Work out the finished part from the listing and answer in its coordinate system (mm). A direction names the side the tool comes from. Round coordinates to 2 decimals unless told otherwise and drop trailing zeros. Loops run counter-clockwise (first coordinate to the right, second up) from the corner with the lowest first, then second, coordinate; pieces in that order, holes last. Notation, with made-up numbers: (28.5, 24) - (40.5, 24) arc R28 ccw to (40.5, 44) - close; hole circle Ø1 at (20.25, 3.5). An arc over 180 degrees is marked (long way). Answer as CSV lines item,"result". Start each with the question number.
Q1. Each of these flat-tipped pins is pushed along its axis until it touches: pin 1 Ø1.1 at (y, z) = (11, -8) entering from +X; pin 2 Ø1.2 at (x, z) = (-1, 6.5) entering from +Y; pin 3 Ø3 at (x, y) = (-4, 1.5) entering from -Z; pin 4 Ø3 at (y, z) = (7.5, 3) entering from +X. Where does it stop, or does it pass through?
Q2. Section C-C on z = -6.5 is taken. Write down the section's boundary in (x, y).
Q3. Section A-A on y = 10.5 is taken. Write down the section's boundary in (x, z).
Q4. For faces 4 (the face through (0, 1.5, 0)), 5 (the face through (-2.663, 11, -7)), 6 (the face through (-2, 9.5, -11)), 7 (the face through (-1, 11, 10)), determine the directions among +Z, -Z, +X, -X, +Y, -Y from which every point of the face is accessible in a straight line to the end or side of a thin tool.
Q5. Section D-D on y = 4.5 is taken. Write down the section's boundary in (x, z), then the cut area to 3 significant figures.
Q6. Straight lines are drawn through the part: L1, parallel to Z at x = 1, y = 7; L2, parallel to X at y = 11.75, z = -7; L3, parallel to Y at x = 4.75, z = 4.5. For each, find the intervals that lie inside material, in ascending order. Write a range as [from, to].
Q7. The mould has two halves that part along X. Classify faces 1 (the face through (-1.5, 11, 12.5)), 2 (the face through (-1, 9.5, -7)), 3 (the face through (-6, 1, 1)): +X half, -X half, draft (parallel to the pull), parting line (faces both ways), or undercut.
Q8. Section B-B on x = -1.5 is taken. Write down the section's boundary in (y, z), then the cut area to 3 significant figures.
```python
from build123d import *

# Parameters (mm, degrees)
SKETCH_1_W               = 12
SKETCH_1_H               = 15
EXTRUDE_1_DEPTH          = 1.5
SKETCH_2_W               = 12
SKETCH_2_H               = 1.5
EXTRUDE_2_DEPTH          = 11
SKETCH_3_W               = 9
SKETCH_3_H               = 6.5
EXTRUDE_3_DEPTH          = 3
FILLET_1_R               = 4
CUT_EXTRUDE_1_DEPTH      = 19.668154703
CUT_EXTRUDE_1_DEPTH_BACK = 3
FILLET_2_R               = 4


with BuildPart() as part:
    # 草图1 → 凸台-拉伸1 (new body)
    with BuildSketch(Plane(origin=(0, 0, 0), x_dir=(1, 0, 0), z_dir=(0, 1, 0))):
        Rectangle(SKETCH_1_W, SKETCH_1_H)
    extrude(amount=EXTRUDE_1_DEPTH)

    # 草图2 → 凸台-拉伸2 (add)
    with BuildSketch(Plane(origin=(0, 1.5, 0), x_dir=(1, 0, 0), z_dir=(0, 1, 0))):
        with Locations((0, 6.75)):
            Rectangle(SKETCH_2_W, SKETCH_2_H)
        with Locations((0, -6.75)):
            Rectangle(SKETCH_2_W, SKETCH_2_H)
    extrude(amount=EXTRUDE_2_DEPTH)

    # 草图3 → 凸台-拉伸3 (add)
    with BuildSketch(Plane(origin=(0, 12.5, 0), x_dir=(1, 0, 0), z_dir=(0, 1, 0))):
        with Locations((-1.5, 9.25)):
            Rectangle(SKETCH_3_W, SKETCH_3_H)
        with Locations((-1.5, -9.25)):
            Rectangle(SKETCH_3_W, SKETCH_3_H)
    extrude(amount=-EXTRUDE_3_DEPTH)

    # 圆角1
    fillet_1_edges = [part.edges().sort_by_distance(p)[0] for p in [
        (3, 11, -12.5),
        (-6, 11, -12.5),
    ]]
    fillet(fillet_1_edges, radius=FILLET_1_R)

    # 草图4 → 切除-拉伸1 (cut, two sides: drawn at the far end of the back side and taken through both)
    with BuildSketch(Plane(origin=(0, 12.5, 0), x_dir=(1, 0, 0), z_dir=(0, 1, 0)).offset(-CUT_EXTRUDE_1_DEPTH_BACK)):
        with BuildLine():
            Line((-2.66316567, 8.819250258), (-2.66316567, 6))
            Line((-2.66316567, 6), (-0.16316567, 6))
            Line((-0.16316567, 6), (-0.16316567, 8.819250258))
            ThreePointArc((-0.16316567, 8.819250258), (-1.41316567, 10.069250258), (-2.66316567, 8.819250258))
        make_face()
        with BuildLine():
            Line((-0.16316567, -6), (-0.16316567, -8.819250258))
            ThreePointArc((-0.16316567, -8.819250258), (-1.41316567, -10.069250258), (-2.66316567, -8.819250258))
            Line((-2.66316567, -8.819250258), (-2.66316567, -6))
            Line((-2.66316567, -6), (-0.16316567, -6))
        make_face()
    extrude(amount=CUT_EXTRUDE_1_DEPTH + CUT_EXTRUDE_1_DEPTH_BACK, mode=Mode.SUBTRACT)

    # 圆角2
    fillet_2_edges = [part.edges().sort_by_distance(p)[0] for p in [
        (-6, 11, 12.5),
        (3, 11, 12.5),
    ]]
    fillet(fillet_2_edges, radius=FILLET_2_R)


solid = part.part
```
Findings:
1,pin 1,"stops at x = 6"
1,pin 2,"stops at y = 9.5"
1,pin 3,"stops at z = -7.5"
1,pin 4,"passes through"
2,outline,"(-6, 0) - (6, 0) - (6, 12.5) - (-0.16, 12.5) - (-0.16, 9.5) - (-2.66, 9.5) - (-2.66, 12.5) - (-6, 12.5) - close"
3,outline,"(-6, -8.5) arc R4 ccw to (-2, -12.5) - (-1, -12.5) arc R4 ccw to (3, -8.5) - (3, -7.5) - (6, -7.5) - (6, -6) - (-0.16, -6) - (-0.16, -8.82) arc R1.25 cw to (-2.66, -8.82) - (-2.66, -6) - (-6, -6) - close; (-6, 6) - (-2.66, 6) - (-2.66, 8.82) arc R1.25 cw to (-0.16, 8.82) - (-0.16, 6) - (6, 6) - (6, 7.5) - (3, 7.5) - (3, 8.5) arc R4 ccw to (-1, 12.5) - (-2, 12.5) arc R4 ccw to (-6, 8.5) - close"
4,face 4,"+X, -X, +Y"
4,face 5,"+Y"
4,face 6,"-Z, +X, -X, -Y"
4,face 7,"+Y, -Y"
5,outline,"(-6, -7.5) - (6, -7.5) - (6, -6) - (-6, -6) - close; (-6, 6) - (6, 6) - (6, 7.5) - (-6, 7.5) - close"
5,area,"36.0 mm^2"
6,L1,"z = [-7.5, -6], [6, 7.5]"
6,L2,"x = [-6, -2.66], [-0.16, 6]"
6,L3,"y = [0, 1.5]"
7,face 1,"draft"
7,face 2,"undercut"
7,face 3,"-X half"
8,outline,"(0, -7.5) - (9.5, -7.5) - (9.5, -6) - (1.5, -6) - (1.5, 6) - (9.5, 6) - (9.5, 7.5) - (0, 7.5) - close; (9.5, -12.5) - (12.5, -12.5) - (12.5, -10.07) - (9.5, -10.07) - close; (9.5, 10.07) - (12.5, 10.07) - (12.5, 12.5) - (9.5, 12.5) - close"
8,area,"61.1 mm^2"
